Print and shaded views of the part. All mm, measured from the part's lowest x, y and z. Give positions to 0.01 mm unless a question says otherwise; leave off trailing zeros. Loops run counter-clockwise (first coordinate to the right, second up) from the corner with the lowest first, then second, coordinate; pieces in that order, holes last.
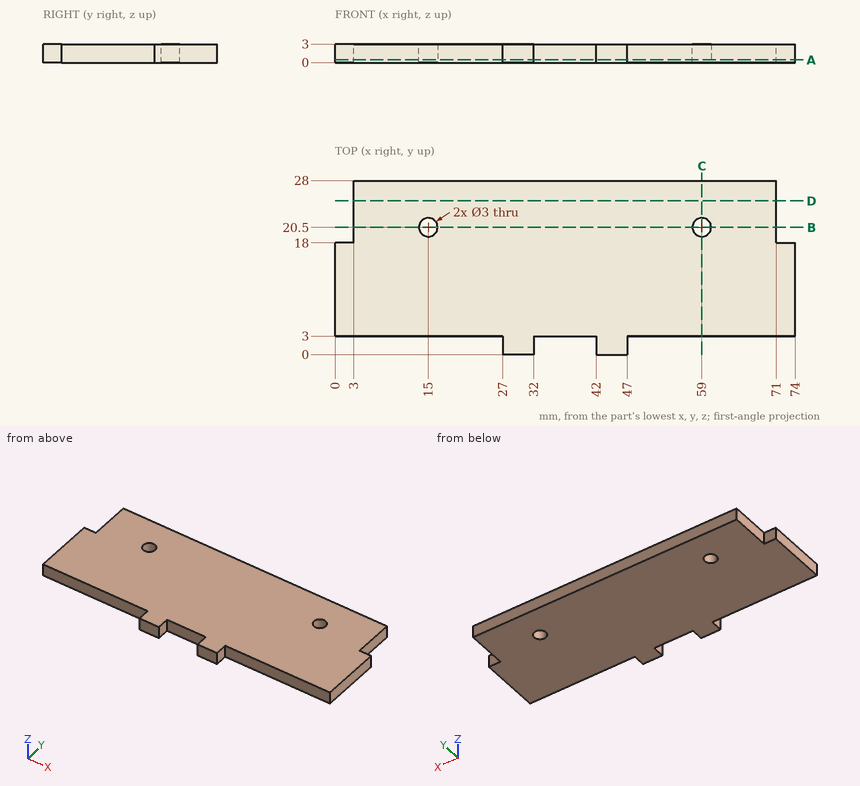
1. Saw through at D-D, the plane y = 24.75. List the corners of the cut face in (x, z).
Responses:
outline: (3, 0) - (71, 0) - (71, 3) - (3, 3) - close
2. Saw through at A-A, the plane z = 0.45. List the corners of the cut face in (x, y), and give its area (3 significant figures).
Responses:
outline: (0, 3) - (27, 3) - (27, 0) - (32, 0) - (32, 3) - (42, 3) - (42, 0) - (47, 0) - (47, 3) - (74, 3) - (74, 18) - (71, 18) - (71, 28) - (3, 28) - (3, 18) - (0, 18) - close; hole circle Ø3 at (15, 20.5); hole circle Ø3 at (59, 20.5)
area: 1,810 mm2
3. Drop flat-ended pins along their axis: pin 1 (1.5 mm diameter, centred on y = 25.5, z = 2, fed in from +X); pin 2 (1.5 mm diameter, centred on x = 36.5, z = 1.5, fed in from -Y); pin 3 (0.9 mm diameter, centred on y = 1, z = 1.5, fed in from -X). Give the stop position or say it passes through.
Responses:
pin 1: stops at x = 71
pin 2: stops at y = 3
pin 3: stops at x = 27
4. Probe line 1 along Y through (x, z) = (59, 1.8); line 2 along X through (y, z) = (22.5, 1.95); line 3 along X through (y, z) = (1.5, 0.7). List the from-to ranges inside material, lowest first.
Responses:
line 1: y = 3 to 19, 22 to 28
line 2: x = 3 to 71
line 3: x = 27 to 32, 42 to 47
5. Saw through at B-B, the plane y = 20.5. List the corners of the cut face in (x, z), and give its area (3 significant figures).
Responses:
outline: (3, 0) - (13.5, 0) - (13.5, 3) - (3, 3) - close; (16.5, 0) - (57.5, 0) - (57.5, 3) - (16.5, 3) - close; (60.5, 0) - (71, 0) - (71, 3) - (60.5, 3) - close
area: 186 mm2
6. Saw through at C-C, the plane x = 59. List the corners of the cut face in (y, z), and give its area (3 significant figures).
Responses:
outline: (3, 0) - (19, 0) - (19, 3) - (3, 3) - close; (22, 0) - (28, 0) - (28, 3) - (22, 3) - close
area: 66.0 mm2
